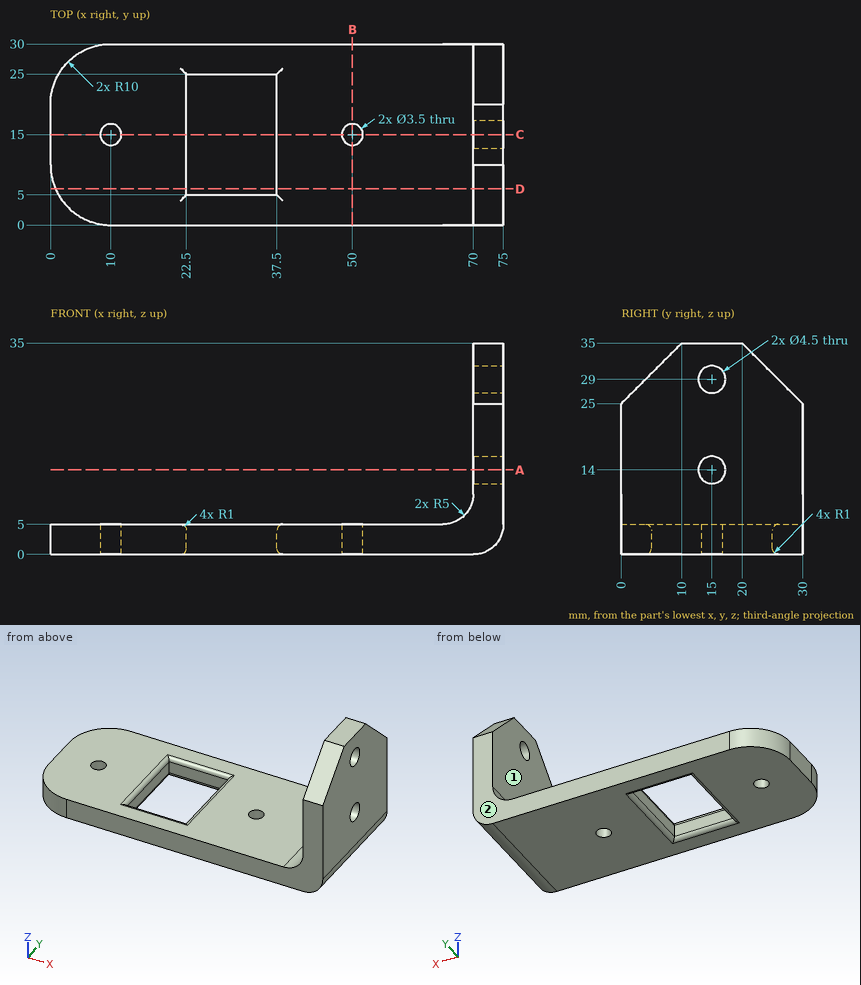
Geometry: see drawing. Coordinates: mm, zero at the bounding-box minimum. A direction names the side the tool comes from. Coordinates: 2 decimals unless noted, no trailing zeros. Write each loop counter-clockwise with the first axis right and the second up, starting at its lowest first coordinate (ties: lowest second). Pieces come first, ordered by that corner, then holes.
1) Set-up query: the marked faces 1 and 2. Return all of +Z, -Z, +X, -X, +Y, -Y with unobstructed straight access to the full face (end or side cutting, diameter ignored); none if empty.
2) Material intervals for line 1 along Y through (x, z) = (10, 3.7); line 2 along Z through (x, y) = (71.9, 15); line 3 along Z through (x, y) = (14.5, 15), sorted ascending.
3) Section B-B on x = 50. Output: boundary loops of the cut face in (y, z).
4) Section C-C on y = 15. State how many separate pieces and enclosed holes the cut face has, and give its area (3 significant figures).
5) Section A-A on z = 14. Output: boundary loops of the cut face in (x, y).
6) Section D-D on y = 6. Output: boundary loops of the cut face in (x, z), and give its area (3 significant figures).
7) Pin query (flat end, axial travel): pin 1 Ø15 at (x, y) = (18, 20.5) entering from +Z; pin 2 Ø3 at (y, z) = (24.5, 23.5) entering from -X; pin 3 Ø2.5 at (y, z) = (18.5, 3) entering from +X. Return the tip coordinate at first contact, or that it passes through.
Check result:
1. face 1: +Z, -X, +Y, -Y
1. face 2: +Z, -Z, +X, -X, +Y
2. line 1: y = 0 to 13.25, 16.75 to 30
2. line 2: z = 0.38 to 11.75, 16.25 to 26.75, 31.25 to 35
2. line 3: z = 0 to 5
3. outline: (0, 0) - (13.25, 0) - (13.25, 5) - (0, 5) - close; (16.75, 0) - (30, 0) - (30, 5) - (16.75, 5) - close
4. separate pieces: 6
4. enclosed holes: 0
4. area: 369 mm2
5. outline: (70, 0) - (75, 0) - (75, 12.75) - (70, 12.75) - close; (70, 17.25) - (75, 17.25) - (75, 30) - (70, 30) - close
6. outline: (0.83, 0) - (21.5, 0) arc R1 ccw to (22.5, 1) - (22.5, 4) arc R1 ccw to (21.5, 5) - (0.83, 5) - close; (37.5, 1) arc R1 ccw to (38.5, 0) - (70, 0) arc R5 ccw to (75, 5) - (75, 31) - (70, 31) - (70, 10) arc R5 cw to (65, 5) - (38.5, 5) arc R1 ccw to (37.5, 4) - close
6. area: 425 mm2
7. pin 1: stops at z = 5
7. pin 2: stops at x = 70
7. pin 3: stops at x = 74.94
